The model under review builds one solid part; all positions refer to its coordinate system, in mm. Face numbers are marked on the shaded views. A direction names the side the tool comes from. Give positions to 0.01 mm unless a question says otherwise; leave off trailing zeros. Write each question's results on one line, items separated by ' | '. Start each with the question number.
Q1. Mouldability with a two-part tool opening along Y and no side actions: class the marked faces 1 and 2 as released by +Y, released by -Y, zero draft, split by the parting line, or undercut.
Q2. Machinability: for the marked faces 3 and 4, which of the approach directions +Z, -Z, +X, -X, +Y, -Y give a long, thin tool a straight path to every point of the face, cutting with its end or side? Answer none if there is none.
Q3. Wall thickness on L1, parallel to Y at x = -1, z = 1.5; L2, parallel to Y at x = 8, z = -7.5; L3, parallel to Z at x = -16, y = 11: over which ranges is each line inside the solid? List them lowest first. Write a range as [from, to].
Q4. Insertion check: pin 1 Ø5 at (x, z) = (7, 1.5) entering from +Y; pin 2 Ø0.5 at (x, z) = (18, -3.5) entering from -Y; pin 3 Ø1.2 at (x, z) = (-18.5, 2.5) entering from +Y. Each pin has a flat end and moves straight along its axis. Give the tip position at first contact, or say it passes through.
from build123d import *

# Parameters (mm, degrees)
SKETCH_1_R               = 27
EXTRUDE_1_DEPTH          = 10
FILLET_1_R               = 2
SKETCH_3_R               = 17.5
CUT_EXTRUDE_1_DEPTH      = 9
SKETCH_5_R               = 15.5
CUT_EXTRUDE_2_DEPTH      = 44.10452425
CUT_EXTRUDE_3_DEPTH      = 9
PATTERN_CIRCULAR_1_COUNT = 12
CUT_EXTRUDE_START        = -4
SKETCH_7_R               = 30.427908266
SKETCH_7_R_2             = 26
CUT_EXTRUDE_4_DEPTH      = 2.4
PATTERN_LINEAR_1_COUNT   = 3
PATTERN_LINEAR_1_PITCH   = 4.8


with BuildPart() as part:
    # 草图1 → 凸台-拉伸1 (new, symmetric)
    with BuildSketch(Plane.XY):
        Circle(SKETCH_1_R)
    extrude(amount=EXTRUDE_1_DEPTH, both=True)

    # 圆角1
    fillet_1_edges = [part.edges().sort_by_distance(p)[0] for p in [
        (-27, 0, -10),
        (-27, 0, 10),
    ]]
    fillet(fillet_1_edges, radius=FILLET_1_R)

    # 草图3 → 切除-拉伸1 (cut, symmetric)
    with BuildSketch(Plane.XY):
        Circle(SKETCH_3_R)
    extrude(amount=CUT_EXTRUDE_1_DEPTH, both=True, mode=Mode.SUBTRACT)

    # 草图5 → 切除-拉伸2 (cut, through all)
    with BuildSketch(Plane.XY.offset(10)):
        Circle(SKETCH_5_R)
    extrude(amount=-CUT_EXTRUDE_2_DEPTH, mode=Mode.SUBTRACT)

    # 草图6 → 切除-拉伸3 (cut, symmetric)
    with BuildSketch(Plane.XY):
        with BuildLine():
            Line((0.5, 17.492855685), (0.5, 19))
            Line((0.5, 19), (2, 19))
            Line((2, 19), (2, 20))
            Line((2, 20), (-2, 20))
            Line((-2, 20), (-2, 19))
            Line((-2, 19), (-0.5, 19))
            Line((-0.5, 19), (-0.5, 17.492855685))
            ThreePointArc((-0.5, 17.492855685), (0, 17.5), (0.5, 17.492855685))
        make_face()
    cut_extrude_3 = extrude(amount=CUT_EXTRUDE_3_DEPTH, both=True, mode=Mode.SUBTRACT)

    # 阵列(圆周)1: 切除-拉伸3 ×12 about axis
    pattern_circular_1_axis = Axis((0, 0, 0), (0, 0, 1))
    for i in range(1, PATTERN_CIRCULAR_1_COUNT):
        add(cut_extrude_3.rotate(pattern_circular_1_axis, i * 360 / PATTERN_CIRCULAR_1_COUNT), mode=Mode.SUBTRACT)

    # 草图7 → 切除-拉伸4 (cut)
    with BuildSketch(Plane(origin=(0, 0, -10), x_dir=(-1, 0, 0), z_dir=(0, 0, -1)).offset(CUT_EXTRUDE_START)):
        Circle(SKETCH_7_R)
        Circle(SKETCH_7_R_2, mode=Mode.SUBTRACT)
    cut_extrude_4 = extrude(amount=-CUT_EXTRUDE_4_DEPTH, mode=Mode.SUBTRACT)

    # 阵列(线性)1: 切除-拉伸4 ×3
    with Locations(*[(0, 0, i * PATTERN_LINEAR_1_PITCH) for i in range(1, PATTERN_LINEAR_1_COUNT)]):
        add(cut_extrude_4, mode=Mode.SUBTRACT)


solid = part.part
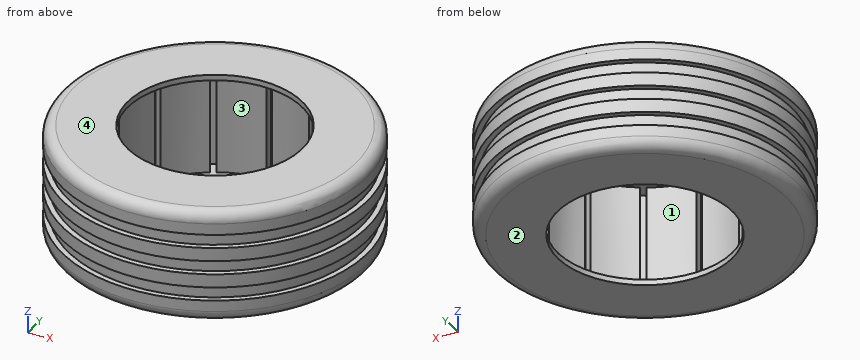
Output:
1) face 1: undercut | face 2: zero draft
2) face 3: none | face 4: +Z, +X, -X, +Y, -Y
3) L1: [-26.98, -20], [-19, -17.47], [17.47, 19], [20, 26.98] | L2: [-25.79, -17.86], [-17.32, -15.56], [15.56, 17.32], [17.86, 25.79] | L3: [-10, -9], [9, 10]
4) pin 1: y = 26.62 | pin 2: y = -20.35 | pin 3: y = 20.21
